Model file for the job. Use its own axes, mm. A direction names the side the tool comes from. Coordinates: 2 decimals unless noted, no trailing zeros. Loops run counter-clockwise (first coordinate to the right, second up) from the corner with the lowest first, then second, coordinate; pieces in that order, holes last. Notation, with made-up numbers: (80.5, 75) -> (126.5, 75) arc R25 ccw to (126.5, 102) -> close; hole circle Ø10 at (37.5, 19.25). An arc over 180 degrees is marked (long way). Use one line per item in the form item = value.
```python
from build123d import *

# Parameters (mm, degrees)
IZIM2_R                          = 15
IZIM2_R_2                        = 10
Y_KSEKLIK_EKSTR_ZYON1_DEPTH      = 12.05
IZIM3_R                          = 10
Y_KSEKLIK_EKSTR_ZYON2_DEPTH      = 5
IZIM4_R                          = 15
Y_KSEKLIK_EKSTR_ZYON3_DEPTH      = 5
IZIM7_R                          = 15
IZIM7_R_2                        = 10
Y_KSEKLIK_EKSTR_ZYON4_DEPTH      = 5
IZIM5_R                          = 5.907014981
Y_KSEKLIK_EKSTR_ZYON5_DEPTH      = 1
Y_KSEKLIK_EKSTR_ZYON5_DEPTH_BACK = 35


with BuildPart() as part:
    # izim2 → Y_kseklik-Ekstr_zyon1 (new body, symmetric)
    with BuildSketch(Plane(origin=(0, 0, 0), x_dir=(0, 0, -1), z_dir=(1, 0, 0))):
        Circle(IZIM2_R)
        Circle(IZIM2_R_2, mode=Mode.SUBTRACT)
    extrude(amount=Y_KSEKLIK_EKSTR_ZYON1_DEPTH, both=True)

    # izim3 → Y_kseklik-Ekstr_zyon2 (add)
    with BuildSketch(Plane(origin=(12.05, 0, 0), x_dir=(0, 0, -1), z_dir=(1, 0, 0))):
        with BuildLine():
            Line((-4, 42.176870951), (4, 42.176870951))
            Line((4, 42.176870951), (17.395555059, 28.781315891))
            Line((17.395555059, 28.781315891), (22.914530919, -14.80525669))
            ThreePointArc((22.914530919, -14.80525669), (0, -26.990652818), (-22.914530919, -14.80525669))
            Line((-22.914530919, -14.80525669), (-17.395555059, 28.781315891))
            Line((-17.395555059, 28.781315891), (-4, 42.176870951))
        make_face()
        Circle(IZIM3_R, mode=Mode.SUBTRACT)
    extrude(amount=Y_KSEKLIK_EKSTR_ZYON2_DEPTH)



with BuildPart() as body_2:
    # izim4 → Y_kseklik-Ekstr_zyon3 (new body)
    with BuildSketch(Plane.ZY.offset(12.05)):
        with BuildLine():
            Line((-4, 42.176870951), (4, 42.176870951))
            Line((4, 42.176870951), (17.395555059, 28.781315891))
            Line((17.395555059, 28.781315891), (22.914530919, -14.80525669))
            ThreePointArc((22.914530919, -14.80525669), (0, -26.990652818), (-22.914530919, -14.80525669))
            Line((-22.914530919, -14.80525669), (-17.395555059, 28.781315891))
            Line((-17.395555059, 28.781315891), (-4, 42.176870951))
        make_face()
        Circle(IZIM4_R, mode=Mode.SUBTRACT)
    extrude(amount=Y_KSEKLIK_EKSTR_ZYON3_DEPTH)


with BuildPart() as part_1:
    add(part.part)

    add(body_2.part)  # Y_kseklik-Ekstr_zyon4 merges body 2
    # izim7 → Y_kseklik-Ekstr_zyon4 (add)
    with BuildSketch(Plane.ZY.offset(12.05)):
        Circle(IZIM7_R)
        Circle(IZIM7_R_2, mode=Mode.SUBTRACT)
    extrude(amount=Y_KSEKLIK_EKSTR_ZYON4_DEPTH)

    # izim5 → Y_kseklik-Ekstr_zyon5 (add, two sides)
    with BuildSketch(Plane.ZY.offset(17.05)) as y_kseklik_ekstr_zyon5_sk:
        with Locations((0, 32.957419359)):
            Circle(IZIM5_R)
    extrude(amount=Y_KSEKLIK_EKSTR_ZYON5_DEPTH)
    extrude(y_kseklik_ekstr_zyon5_sk.sketch, amount=-Y_KSEKLIK_EKSTR_ZYON5_DEPTH_BACK)


solid = part_1.part
```
Q1. Band-saw the part on A-A, the plane z = 0. Write the cut outline in (x, y).
Result:
outline = (-18.05, 27.05) -> (-17.05, 27.05) -> (-17.05, 10) -> (17.05, 10) -> (17.05, 27.05) -> (17.95, 27.05) -> (17.95, 38.86) -> (17.05, 38.86) -> (17.05, 42.18) -> (12.05, 42.18) -> (12.05, 38.86) -> (-12.05, 38.86) -> (-12.05, 42.18) -> (-17.05, 42.18) -> (-17.05, 38.86) -> (-18.05, 38.86) -> close; (-17.05, -26.99) -> (-12.05, -26.99) -> (-12.05, -15) -> (12.05, -15) -> (12.05, -26.99) -> (17.05, -26.99) -> (17.05, -10) -> (-17.05, -10) -> close; hole (-12.05, 15) -> (12.05, 15) -> (12.05, 27.05) -> (-12.05, 27.05) -> close
Q2. Wall check: line 1 along Y through (x, z) = (-3, 0); line 2 along X through (y, z) = (-21.5, 7.5); line 3 along Z through (x, y) = (8, 0). Give the ranges that are in metal, low to high.
Result:
line_1 = -15 to -10, 10 to 15, 27.05 to 38.86
line_2 = -17.05 to -12.05, 12.05 to 17.05
line_3 = -15 to -10, 10 to 15
Q3. Pin check, flat tips, straight feed: pin 1 Ø3 at (y, z) = (25, 5) entering from +X; pin 2 Ø10 at (x, z) = (-5, 16) entering from -Y; pin 3 Ø16 at (y, z) = (0, 0) entering from -X; pin 4 Ø8 at (x, y) = (7.5, -1) entering from +Z. Stop position of each tip, or through.
Result:
pin_1 = 17.05
pin_2 = -10.2
pin_3 = through
pin_4 = 15
Q4. Band-saw the part on B-B, the plane y = 2.5. Write the cut outline in (x, z), and give its area (3 significant figures).
Result:
outline = (-17.05, -20.72) -> (-12.05, -20.72) -> (-12.05, -14.79) -> (12.05, -14.79) -> (12.05, -20.72) -> (17.05, -20.72) -> (17.05, -9.68) -> (-17.05, -9.68) -> close; (-17.05, 9.68) -> (17.05, 9.68) -> (17.05, 20.72) -> (12.05, 20.72) -> (12.05, 14.79) -> (-12.05, 14.79) -> (-12.05, 20.72) -> (-17.05, 20.72) -> close
area = 467 mm2
Q5. Band-saw the part on D-D, the plane z = -8. Write the cut outline in (x, y), and give its area (3 significant figures).
Result:
outline = (-17.05, -25.81) -> (-12.05, -25.81) -> (-12.05, -12.69) -> (12.05, -12.69) -> (12.05, -25.81) -> (17.05, -25.81) -> (17.05, -6) -> (-17.05, -6) -> close; (-17.05, 6) -> (17.05, 6) -> (17.05, 38.18) -> (12.05, 38.18) -> (12.05, 12.69) -> (-12.05, 12.69) -> (-12.05, 38.18) -> (-17.05, 38.18) -> close
area = 842 mm2
Q6. Which spindle directions (+Z, -Z, +X, -X, +Y, -Y) get a long thin tool onto all of the face, cutting with end or side? Do faces 1 (the face through (14.515, 7.293, -20.116)), 2 (the face through (-0.17, 27.19, -1.28)), 3 (the face through (-17.54, 27.19, -1.28)), 4 (the face through (17.49, 27.19, -1.28)), 5 (the face through (15, 42.177, 0)). Say none if no direction does.
Result:
face_1 = -Z, +X, -X, +Y
face_2 = none
face_3 = -X
face_4 = +X
face_5 = +Z, -Z, +X, -X, +Y
Q7. Mould opens along X. For faces 6 (the face through (14.515, 35.573, -10.604)), 7 (the face through (-12.05, 16, 0)), 8 (the face through (17.05, 0, -11)), 9 (the face through (-18.05, 33, 0)) say: released by +X, released by -X, zero draft, split by the parting line, or undercut.
Result:
face_6 = zero draft
face_7 = undercut
face_8 = released by +X
face_9 = released by -X
Q8. Band-saw the part on C-C, the plane x = 13.5. Write the cut outline in (y, z), and give its area (3 significant figures).
Result:
outline = (-14.81, -22.91) -> (28.78, -17.4) -> (42.18, -4) -> (42.18, 4) -> (28.78, 17.4) -> (-14.81, 22.91) arc R27.64 ccw to start; hole circle Ø20 at (0, 0)
area = 2,120 mm2
